```python
from build123d import *

# Parameters (mm, degrees)
F1_DEPTH = 15
F2_W     = 19
F2_H     = 8
F3_DEPTH = 6
F5_DEPTH = 2
F6_R     = 3


with BuildPart() as f1:
    # F0 (on Front) → F1 (new body)
    with BuildSketch(Plane.XZ):
        Polygon((24, -20.78461), (18, -10.392305), (12, -20.78461), (-12, -20.78461), (-18, -10.392305), (-24, -20.78461), (-12, -41.569219), (12, -41.569219), align=None)
        Polygon((12, -20.78461), (18, -10.392305), (12, 0), (6, -10.392305), (-6, -10.392305), (-12, 0), (-18, -10.392305), (-12, -20.78461), align=None)
        Polygon((-12, 0), (-12, 20.78461), (-24, 0), (-18, -10.392305), align=None)
        Polygon((18, -10.392305), (24, 0), (12, 20.78461), (12, 0), align=None)
        with BuildLine():
            Line((-24, 0), (-12, 20.78461))
            ThreePointArc((-12, 20.78461), (-20.78461, 12), (-24, 0))
        make_face()
        with BuildLine():
            Line((12, 20.78461), (24, 0))
            ThreePointArc((24, 0), (20.78461, 12), (12, 20.78461))
        make_face()
        Polygon((24, -20.78461), (24, 0), (18, -10.392305), align=None)
        Polygon((-18, -10.392305), (-24, 0), (-24, -20.78461), align=None)
    extrude(amount=F1_DEPTH)

    # F2 (on face) → F3 (cut)
    with BuildSketch(Plane(origin=(0, 0, -41.569219), x_dir=(1, 0, 0), z_dir=(0, 0, -1))):
        with Locations((0, 7.5)):
            Rectangle(F2_W, F2_H)
    extrude(amount=-F3_DEPTH, mode=Mode.SUBTRACT)

    # F4 (on face) → F5 (join)
    with BuildSketch(Plane.XZ.offset(15)):
        with BuildLine():
            ThreePointArc((-24, 0), (0, -24), (24, 0))
            ThreePointArc((24, 0), (0, 24), (-24, 0))
        make_face()
        with BuildLine():
            Line((24, -20.78461), (24, 0))
            ThreePointArc((24, 0), (0, -24), (-24, 0))
            Line((-24, 0), (-24, -20.78461))
            Line((-24, -20.78461), (-12, -41.569219))
            Line((-12, -41.569219), (12, -41.569219))
            Line((12, -41.569219), (24, -20.78461))
        make_face()
    extrude(amount=F5_DEPTH)

    # F6
    f6_edges = [f1.edges().sort_by_distance(p)[0] for p in [
        (0, -3.5, -35.569219),
        (-9.5, -7.5, -35.569219),
        (0, -11.5, -35.569219),
        (9.5, -7.5, -35.569219),
    ]]
    fillet(f6_edges, radius=F6_R)


solid = f1.part
```
Input: part model. Units: mm. Frame: model coordinates. A direction names the side the tool comes from. Give positions to 0.01 mm unless a question says otherwise; leave off trailing zeros. Loops run counter-clockwise (first coordinate to the right, second up) from the corner with the lowest first, then second, coordinate; pieces in that order, holes last.
1) Section query C-C on y = -2. Return the cut outline in (x, z).
A:
outline: (-24, -20.78) - (-12, -41.57) - (12, -41.57) - (24, -20.78) - (24, 0) arc R24 ccw to (12, 20.78) - (12, 0) - (6, -10.39) - (-6, -10.39) - (-12, 0) - (-12, 20.78) arc R24 ccw to (-24, 0) - close
2) Line query: L1, parallel to Y at x = 6.5, z = 5; L2, parallel to X at y = -7.25, z = 6.5; L3, parallel to X at y = -7.5, z = -2.5. Output: solid intervals per line, ascending.
A:
L1: y = -17 to -15
L2: x = -23.1 to -12, 12 to 23.1
L3: x = -24 to -10.56, 10.56 to 24
3) Section query D-D on z = 9. Return the cut outline in (x, y), and give its area (3 significant figures).
A:
outline: (-22.25, -17) - (22.25, -17) - (22.25, 0) - (12, 0) - (12, -15) - (-12, -15) - (-12, 0) - (-22.25, 0) - close
area: 396 mm2
4) Contact query for flat-ended pins moving along their axis: pin 1 (3 mm diameter, centred on x = 14.5, z = -13, fed in from +Y); pin 2 (8 mm diameter, centred on x = 6.5, z = 17, fed in from +Y); pin 3 (4 mm diameter, centred on x = 17, y = -5, fed in from -Z); pin 4 (1.5 mm diameter, centred on y = -8, z = -39.5, fed in from +X). Output: stop coordinate, or through.
A:
pin 1: stops at y = 0
pin 2: stops at y = -15
pin 3: stops at z = -36.37
pin 4: stops at x = 13.63
5) Mould query, pull axis X, two halves, no side actions, for faces 1 (the cylindrical face through (0.133, -10.598, -36.425)), 2 (the flat face through (0, -17, -8)), 3 (the flat face through (24, -8, -11)), 4 (the cylindrical face through (-8.98, -7.56, -36.88)). Classes: released by +X, released by -X, zero draft, split by the parting line, or undercut.
A:
face 1: undercut
face 2: zero draft
face 3: released by +X
face 4: undercut
6) Section query B-B on x = 0. Return the cut outline in (y, z).
A:
outline: (-17, -41.57) - (-11.5, -41.57) - (-11.5, -38.57) arc R3 cw to (-8.5, -35.57) - (-6.5, -35.57) arc R3 cw to (-3.5, -38.57) - (-3.5, -41.57) - (0, -41.57) - (0, -10.39) - (-15, -10.39) - (-15, 24) - (-17, 24) - close
7) Reachability of faces 5 (the flat face through (9.042, -7.395, -5.123)), 6 (the flat face through (0, -8, -35.569)), 7 (the flat face through (-24, -8, -10)) from +Z, -Z, +X, -X, +Y, -Y: full face, straight path, thin tool, end or side. Return the list, or none.
A:
face 5: +Z, +Y
face 6: -Z
face 7: +Z, -Z, -X, +Y, -Y
8) Section query A-A on z = -37. Return the cut outline in (x, y).
A:
outline: (-14.64, -17) - (14.64, -17) - (14.64, 0) - (-14.64, 0) - close; hole (-9.06, -11.06) - (9.06, -11.06) - (9.06, -3.94) - (-9.06, -3.94) - close
